```python
from build123d import *

# Parameters (mm, degrees)
SKETCH_1_R      = 2.25
SKETCH_1_R_2    = 4.5
SKETCH_1_R_3    = 2
EXTRUDE_1_DEPTH = 4


with BuildPart() as part:
    # 草图1 → 凸台-拉伸1 (new body)
    with BuildSketch(Plane.XY):
        Polygon((0, 4.863043478), (-4, 4.863043478), (-4, 12.863043478), (0, 12.863043478), (0, 22.363043478), (4, 22.363043478), (4, 21.013043478), (6.6, 21.013043478), (6.6, 22.363043478), (8.6, 22.363043478), (8.6, 25.363043478), (6.6, 25.363043478), (6.6, 26.713043478), (4, 26.713043478), (4, 25.363043478), (0, 25.363043478), (0, 31.363043478), (56, 31.363043478), (56, 25.363043478), (52, 25.363043478), (52, 26.713043478), (49.4, 26.713043478), (49.4, 25.363043478), (47.4, 25.363043478), (47.4, 22.363043478), (49.4, 22.363043478), (49.4, 21.013043478), (52, 21.013043478), (52, 22.363043478), (56, 22.363043478), (56, 12.863043478), (60, 12.863043478), (60, 4.863043478), (56, 4.863043478), (56, -4.636956522), (52, -4.636956522), (52, -3.286956522), (49.4, -3.286956522), (49.4, -4.636956522), (47.4, -4.636956522), (47.4, -7.636956522), (49.4, -7.636956522), (49.4, -8.986956522), (52, -8.986956522), (52, -7.636956522), (56, -7.636956522), (56, -17.136956522), (60, -17.136956522), (60, -25.136956522), (56, -25.136956522), (56, -105.136956522), (0, -105.136956522), (0, -25.136956522), (-4, -25.136956522), (-4, -17.136956522), (0, -17.136956522), (0, -7.636956522), (4, -7.636956522), (4, -8.986956522), (6.6, -8.986956522), (6.6, -7.636956522), (8.6, -7.636956522), (8.6, -4.636956522), (6.6, -4.636956522), (6.6, -3.286956522), (4, -3.286956522), (4, -4.636956522), (0, -4.636956522), align=None)
        with Locations((28, 8.863043478)):
            Circle(SKETCH_1_R, mode=Mode.SUBTRACT)
        with Locations((28, -56.136956522)):
            Circle(SKETCH_1_R_2, mode=Mode.SUBTRACT)
        with Locations((8, -56.136956522)):
            Circle(SKETCH_1_R_3, mode=Mode.SUBTRACT)
        with Locations((28, -76.136956522)):
            Circle(SKETCH_1_R_3, mode=Mode.SUBTRACT)
        with Locations((48, -56.136956522)):
            Circle(SKETCH_1_R_3, mode=Mode.SUBTRACT)
        with Locations((48, -96.136956522)):
            Circle(SKETCH_1_R_3, mode=Mode.SUBTRACT)
        with Locations((8, -96.136956522)):
            Circle(SKETCH_1_R_3, mode=Mode.SUBTRACT)
    extrude(amount=EXTRUDE_1_DEPTH)


solid = part.part
```
Here's how the part is built. I have some questions about the finished solid (model axes, mm). A direction names the side the tool comes from. Coordinates: 2 decimals unless noted, no trailing zeros. Loops run counter-clockwise (first coordinate to the right, second up) from the corner with the lowest first, then second, coordinate; pieces in that order, holes last. Notation, with made-up numbers: (-22.75, 45) -> (-2.75, 45) arc R23 cw to (-2.75, 79) -> close; hole circle Ø4 at (46.25, -11). An arc over 180 degrees is marked (long way). Return JSON: item names as keys, results as strings.
1) Will these pins go through, and if not, where does the flat tip stop? pin 1 (1.2 mm diameter, centred on y = -52.5, z = 2, fed in from -X); pin 2 (1 mm diameter, centred on y = -83, z = 1, fed in from +X).
Results below:
{"pin 1": "x = 0", "pin 2": "x = 56"}
2) If we section it at A-A, the plane x = 28: Write out the boundary of the cut face in (y, z).
Results below:
{"outline": "(-105.14, 0) -> (-78.14, 0) -> (-78.14, 4) -> (-105.14, 4) -> close; (-74.14, 0) -> (-60.64, 0) -> (-60.64, 4) -> (-74.14, 4) -> close; (-51.64, 0) -> (6.61, 0) -> (6.61, 4) -> (-51.64, 4) -> close; (11.11, 0) -> (31.36, 0) -> (31.36, 4) -> (11.11, 4) -> close"}
3) Thinking about a two-plate mould opening in Y: for faces 1 (the face through (28, -36, 0)), 2 (the face through (54, -4.637, 2)), 3 (the face through (28, -105.137, 2)), 4 (the face through (-2, -17.137, 2)), which applies, +Y half, -Y half, draft (parallel to the pull), parting line (faces both ways), or undercut?
Results below:
{"face 1": "draft", "face 2": "undercut", "face 3": "-Y half", "face 4": "undercut"}
4) If we section it at B-B, the plane y = -38: Write out the boundary of the cut face in (x, z), then the cut area to 3 significant figures.
Results below:
{"outline": "(0, 0) -> (56, 0) -> (56, 4) -> (0, 4) -> close", "area": "224 mm²"}
5) I need wall thicknesses on line 1 (Y direction, x = 28, z = 2.45); line 2 (Y direction, x = 1, z = 0.35); line 3 (X direction, y = -8, z = 0.7). Which ranges of each line are inside material? Lowest first, please. Write a range as from..to.
Results below:
{"line 1": "-105.14..-78.14, -74.14..-60.64, -51.64..6.61, 11.11..31.36", "line 2": "-105.14..-7.64, -4.64..22.36, 25.36..31.36", "line 3": "0..4, 6.6..49.4, 52..56"}
6) For faces 5 (the face through (60, -21, 2)), 6 (the face through (5, 26.713, 2)), 7 (the face through (8.6, -6, 2)), 8 (the face through (54, 22.363, 2)), which set-ups out of +Z, -Z, +X, -X, +Y, -Y let a thin tool reach every point of the face, with its end or its side?
Results below:
{"face 5": "+Z, -Z, +X, +Y, -Y", "face 6": "+Z, -Z", "face 7": "+Z, -Z, -X", "face 8": "+Z, -Z, +X"}
7) If we section it at C-C, the plane z = 2.4: Count the separate pieces of the cut face and the enclosed holes in it, then the cut area to 3 significant figures.
Results below:
{"separate pieces": "1", "enclosed holes": "7", "area": "7,500 mm²"}
